```python
from build123d import *

# Parameters (mm, degrees)
EXTRUDE_1_DEPTH     = 14.999999999999998
CUT_EXTRUDE_1_DEPTH = 32.759958749611776
CUT_EXTRUDE_2_DEPTH = 5.999999999999998
CUT_EXTRUDE_START   = -2.9999999999999996
CUT_EXTRUDE_3_DEPTH = 2.9999999999999996
CUT_EXTRUDE_START_2 = -3.0000000000000004
CUT_EXTRUDE_4_DEPTH = 3.0000000000000004
CUT_EXTRUDE_5_DEPTH = 10.50007039461797
CUT_EXTRUDE_6_DEPTH = 11.327672160759418
EXTRUDE_2_DEPTH     = 7.968709711177614
EXTRUDE_3_DEPTH     = 3.000000000000002
HOLE_WIZARD_1_D     = 4.2
HOLE_WIZARD_1_DEPTH = 7
HOLE_WIZARD_2_D     = 2.03
HOLE_WIZARD_2_DEPTH = 4
HOLE_WIZARD_3_D     = 2.03
HOLE_WIZARD_3_DEPTH = 4
HOLE_WIZARD_4_D     = 5.05
HOLE_WIZARD_5_D     = 5.02
HOLE_WIZARD_5_DEPTH = 12
FILLET_1_R          = 5.500000000000002
FILLET_2_R          = 8
CHAMFER_1_SIZE      = 0.9999999999999993
FILLET_3_R          = 0.5


with BuildPart() as part:
    # 草图1 → 凸台-拉伸1 (new body)
    with BuildSketch(Plane(origin=(0, 18, 0), x_dir=(1, 0, 0), z_dir=(0, 1, 0))):
        with BuildLine():
            Line((-17.618889211708797, -12.26572898251346), (21.661848401793918, 2.0312902888225244))
            Line((21.661848401793918, 2.0312902888225244), (-10.5, 2.0312902888223876))
            Line((-10.5, 2.0312902888223876), (-21.381110788291235, -1.9291101538684705))
            ThreePointArc((-21.381110788291235, -1.9291101538684705), (-24.668309414322497, -8.978530356482176), (-17.618889211708797, -12.26572898251346))
        make_face()
    extrude(amount=-EXTRUDE_1_DEPTH)

    # 草图2 → 切除-拉伸1 (cut, through all)
    with BuildSketch(Plane(origin=(0, 18, 0), x_dir=(-1, 0, 0), z_dir=(0, 1, 0))):
        Polygon((-21.66184840179392, -2.0312902888223894), (-5.5000000000000036, -2.0312902888223876), (-5.500000000000005, 3.8511414601534057), align=None)
    extrude(amount=-CUT_EXTRUDE_1_DEPTH, mode=Mode.SUBTRACT)

    # 草图3 → 切除-拉伸2 (cut)
    with BuildSketch(Plane(origin=(0, 18, 0), x_dir=(-1, 0, 0), z_dir=(0, 1, 0))):
        with BuildLine():
            Line((20.78257553747125, 3.5735722402438013), (24.563305918164147, 4.949645562601932))
            ThreePointArc((24.563305918164147, 4.949645562601932), (24.047293898775088, 10.191303567012326), (19.3611131717343, 12.59566569299606))
            Line((19.3611131717343, 12.59566569299606), (20.01010960022055, 10.812562660423456))
            ThreePointArc((20.01010960022055, 10.812562660423456), (15.771169677152303, 6.6995195513380725), (20.78257553747125, 3.5735722402438013))
        make_face()
    extrude(amount=-CUT_EXTRUDE_2_DEPTH, mode=Mode.SUBTRACT)

    # 草图4 → 切除-拉伸3 (cut)
    with BuildSketch(Plane.XZ.offset(-12).offset(CUT_EXTRUDE_START)):
        with BuildLine():
            Line((-20.78257553747125, 3.573572240243805), (-18.036485631419698, 2.5740772538221752))
            Line((-18.036485631419698, 2.5740772538221752), (-17.557657430763733, 3.889646922922488))
            ThreePointArc((-17.557657430763733, 3.889646922922488), (-19.134214632183554, 3.365302064053206), (-20.78257553747125, 3.573572240243805))
        make_face()
    extrude(amount=CUT_EXTRUDE_3_DEPTH, mode=Mode.SUBTRACT)

    # 草图5 → 切除-拉伸4 (cut)
    with BuildSketch(Plane.XZ.offset(-3.000000000000001).offset(CUT_EXTRUDE_START_2)):
        with BuildLine():
            Line((-17.258794358827192, 2.29102077914986), (-16.779966158171227, 3.606590448250214))
            Line((-16.779966158171227, 3.606590448250214), (-17.557657430763737, 3.8896469229224904))
            ThreePointArc((-17.557657430763737, 3.8896469229224904), (-15.965242102135065, 8.349612286378331), (-20.01010960022055, 10.81256266042346))
            Line((-20.01010960022055, 10.81256266042346), (-19.3611131717343, 12.59566569299606))
            ThreePointArc((-19.3611131717343, 12.59566569299606), (-24.04729389877508, 10.191303567012337), (-24.56330591816415, 4.94964556260195))
            Line((-24.56330591816415, 4.94964556260195), (-17.258794358827192, 2.29102077914986))
        make_face()
    extrude(amount=CUT_EXTRUDE_4_DEPTH, mode=Mode.SUBTRACT)

    # 草图6 → 切除-拉伸5 (cut)
    with BuildSketch(Plane(origin=(-15.97621882135595, 0, 5.8148681070970145), x_dir=(0.3420201433256677, 0, 0.9396926207859088), z_dir=(-0.9396926207859089, 0, 0.3420201433256677))):
        Polygon((-2.3499999999999055, 3), (-2.349999999999906, 6), (-3.7499999999999933, 6), (-3.749999999999994, 3), align=None)
    extrude(amount=-CUT_EXTRUDE_5_DEPTH, mode=Mode.SUBTRACT)

    # 草图7 → 切除-拉伸6 (cut)
    with BuildSketch(Plane(origin=(-16.753910093948367, 0, 6.097924581769449), x_dir=(0.3420201433256676, 0, 0.9396926207859088), z_dir=(-0.9396926207859088, 0, 0.3420201433256676))):
        Polygon((-3.749999999999993, 12), (-2.3499999999999055, 12), (-2.3499999999999055, 15), (-3.7499999999999933, 15), align=None)
    extrude(amount=-CUT_EXTRUDE_6_DEPTH, mode=Mode.SUBTRACT)

    # 草图8 → 凸台-拉伸2 (add)
    with BuildSketch(Plane(origin=(-8.63e-15, 0, -2.0312902888224325), x_dir=(-1, 0, 5e-17), z_dir=(-5e-17, 0, -1))):
        Polygon((-5.5, 3), (-5.500000000000001, 18), (10.5, 18), (10.5, 3), align=None)
    extrude(amount=EXTRUDE_2_DEPTH)

    # 草图9 → 凸台-拉伸3 (add)
    with BuildSketch(Plane.XZ.offset(-3.000000000000001)):
        with BuildLine():
            Line((-17.618889211708797, 12.26572898251346), (5.499999999999998, 3.8511414601533294))
            Line((5.499999999999998, 3.8511414601533294), (5.5, -10))
            Line((5.5, -10), (-10.5, -10.000000000000002))
            Line((-10.5, -10.000000000000002), (-10.500000000000014, -2.0312902888224262))
            Line((-10.500000000000014, -2.0312902888224262), (-21.381110788291203, 1.9291101538684652))
            ThreePointArc((-21.381110788291203, 1.9291101538684652), (-23.286441520356178, 3.1083268627098155), (-24.563305918164144, 4.94964556260193))
            Line((-24.563305918164144, 4.94964556260193), (-20.78257553747125, 3.573572240243805))
            ThreePointArc((-20.78257553747125, 3.573572240243805), (-15.771169677152304, 6.699519551338072), (-20.01010960022055, 10.81256266042346))
            Line((-20.01010960022055, 10.81256266042346), (-19.361113171734285, 12.595665692996059))
            ThreePointArc((-19.361113171734285, 12.595665692996059), (-18.476617299855562, 12.50137070130135), (-17.618889211708797, 12.26572898251346))
        make_face()
    extrude(amount=EXTRUDE_3_DEPTH)

    # 孔1
    with Locations(Plane(origin=(-5.4e-16, 0, -10.000000000000046), x_dir=(-1, 0, 5e-17), z_dir=(-5e-17, 0, -1))):
        with Locations((4.5, 9)):
            Hole(HOLE_WIZARD_1_D / 2, depth=HOLE_WIZARD_1_DEPTH)

    # 孔2
    with Locations(Plane(origin=(-5.4e-16, 0, -10.000000000000046), x_dir=(-1, 0, 5e-17), z_dir=(-5e-17, 0, -1))):
        with Locations((-0.5, 13)):
            Hole(HOLE_WIZARD_2_D / 2, depth=HOLE_WIZARD_2_DEPTH)

    # 孔3
    with Locations(Plane(origin=(-5.4e-16, 0, -10.000000000000046), x_dir=(-1, 0, 5e-17), z_dir=(-5e-17, 0, -1))):
        with Locations((-0.5, 5)):
            Hole(HOLE_WIZARD_3_D / 2, depth=HOLE_WIZARD_3_DEPTH)

    # 孔4 (through all)
    with Locations(Plane(origin=(0, 18, 0), x_dir=(1, 0, 0), z_dir=(0, 1, 0))):
        with Locations((-2.585532826, -0.941056988)):
            Hole(HOLE_WIZARD_4_D / 2)

    # 孔5
    with Locations(Plane(origin=(0, 12, 0), x_dir=(1, 0, 0), z_dir=(0, 1, 0))):
        with Locations((-19.5, -7.097419568)):
            Hole(HOLE_WIZARD_5_D / 2, depth=HOLE_WIZARD_5_DEPTH)

    # 圆角1
    fillet_1_edges = [part.edges().sort_by_distance(p)[0] for p in [
        (5.500000000000002, 8.999999999999998, 3.8511414601533676),
    ]]
    fillet(fillet_1_edges, radius=FILLET_1_R)

    # 圆角2
    fillet_2_edges = [part.edges().sort_by_distance(p)[0] for p in [
        (-10.50000000000001, 9, -2.031290288822418),
    ]]
    fillet(fillet_2_edges, radius=FILLET_2_R)

    # 倒角1
    chamfer_1_edges = [part.edges().sort_by_distance(p)[0] for p in [
        (-18.47661729985556, -1.33e-15, 12.50137070130135),
        (-23.286441520356178, -1.33e-15, 3.108326862709817),
        (-18.572474820842935, -1.33e-15, 0.9068502628278257),
        (5.499999999999999, -1.33e-15, -5.000000000000032),
        (-7.868889211708797, -1.33e-15, 8.717019198417944),
        (4.505336243589472, 17.999999999999986, 3.15467039993076),
        (4.505336243589466, -1.65e-14, 3.154670399930683),
        (-10.500000000000002, -1.33e-15, -8.816475297250042),
        (-18.57247482084295, 18, 0.9068502628278368),
        (-11.946783645688074, 17.999999999999993, -3.044339103691696),
        (-11.946783645688082, -7.42e-15, -3.0443391036917093),
        (5.4999999999999964, 18, -5.000000000000016),
        (-18.476617299855565, 18, 12.501370701301362),
        (-7.868889211708806, 18, 8.717019198417947),
        (-23.286441520356195, 18, 3.1083268627098226),
        (-10.500000000000009, 18, -8.816475297250054),
    ]]
    chamfer(chamfer_1_edges, length=CHAMFER_1_SIZE)

    # 圆角3
    fillet_3_edges = [part.edges().sort_by_distance(p)[0] for p in [
        (-14.087265614371681, 3.0000000000000004, 1.1366787190484136),
        (-14.087265614371635, 15, 1.1366787190484962),
        (-15.977630804718132, 6.000000000000001, 1.8247153802274876),
        (-12.23539246068994, 6.000000000000001, 1.9525008949379346),
        (-12.23539246068994, 3.0000000000000004, 1.9525008949379348),
        (-12.235392460689857, 15, 1.952500894938097),
        (-12.235392460689857, 12, 1.952500894938097),
    ]]
    fillet(fillet_3_edges, radius=FILLET_3_R)


solid = part.part
```
The model under review builds one solid part; all positions refer to its coordinate system, in mm. A direction names the side the tool comes from. Coordinates: 2 decimals unless noted, no trailing zeros. Order: outer loops, then holes, each group sorted by start corner. A loop starts at its lowest first (then second) coordinate and runs counter-clockwise, first axis right, second up. Notation, with made-up numbers: (23.25, -29) -> (59.25, -29) arc R21 cw to (59.25, -8) -> close; hole circle Ø9 at (45, 45). An arc over 180 degrees is marked (long way). Answer in a Markdown table with one row per item. Add a question column.
Item 1: We need section B-B on x = -4.5. Write out the cut boundary in (y, z), plus the area to 3 significant figures.
Item 2: We need section A-A on y = 10. Write out the cut boundary in (x, z) (3 decimals).
Item 3: Mouldability with a two-part tool opening along X and no side actions: class faces 1 (the flat face through (-17, 12, 6)), 2 (the flat face through (-5, 9, -3)), 3 (the cylindrical face through (-25, 9, 7)), 4 (the cylindrical face through (-11.91, 9.11, -3.1)) as +X half, -X half, draft (parallel to the pull), parting line (faces both ways), or undercut.
Item 4: Machinability: for faces 5 (the flat face through (-10, 0.5, -8.8)), 6 (the flat face through (-10, 17.5, -8.8)), 7 (the cylindrical face through (0.28, 12.01, -7.97)), which of the approach directions +Z, -Z, +X, -X, +Y, -Y give a long, thin tool a straight path to every point of the face, cutting with its end or side? Answer none if there is none.
Item 5: We need section C-C on y = 5. Write out the cut boundary in (x, z) (3 decimals).
Item 6: Clearance check with flat-ended pins moving along their axes: pin 1 (4.5 mm diameter, centred on x = -4, y = 8.5, fed in from -Z); pin 2 (1.9 mm diameter, centred on y = 5.5, z = -9, fed in from -X); pin 3 (1.6 mm diameter, centred on x = 0.5, y = 13, fed in from +Z); pin 4 (3.5 mm diameter, centred on x = -4.5, y = 9, fed in from +Z). State where each tip first meets the part, or that it passes through.
Item 7: To check wall thickness, follow probe 1 along Y at (x, z) = (-15.5, 2.5); probe 2 along Y at (x, z) = (0.5, -7.15) (3 decimals); probe 3 along Y at (x, z) = (-4.5, -4.5). State the ranges of each line that lie inside material, in increasing order.
Item 8: We need section D-D on x = 1. Write out the cut boundary in (y, z), plus the area to 3 significant figures.
Final values:
| question | item | result |
|---|---|---|
| 1 | outline | (0, -10) -> (6.9, -10) -> (6.9, -3) -> (11.1, -3) -> (11.1, -10) -> (18, -10) -> (18, -0.71) -> (0, -0.71) -> close; (0, 2.59) -> (18, 2.59) -> (18, 6.43) -> (17, 7.49) -> (1, 7.49) -> (0, 6.43) -> close |
| 1 | area | 225 mm2 |
| 2 | outline | (-21.381, 1.929) -> (-15.764, -0.115) arc R8 cw to (-10.5, -7.633) -> (-10.5, -10) -> (-6.347, -10) -> (-6.347, -3) -> (-2.653, -3) -> (-2.653, -10) -> (5.5, -10) -> (5.5, 0) arc R5.5 ccw to (1.881, 5.168) -> (-17.619, 12.266) arc R5.5 ccw to start; hole circle Ø5.02 at (-19.5, 7.097); hole circle Ø5.05 at (-2.586, 0.941) |
| 3 | face 1 | undercut |
| 3 | face 2 | undercut |
| 3 | face 3 | parting line |
| 3 | face 4 | -X half |
| 4 | face 5 | -Z, -X, -Y |
| 4 | face 6 | -Z, -X, +Y |
| 4 | face 7 | -Z |
| 5 | outline | (-24.563, 4.95) arc R5.5 ccw to (-21.381, 1.929) -> (-15.764, -0.115) arc R8 cw to (-10.5, -7.633) -> (-10.5, -10) -> (-0.515, -10) -> (-0.515, -6) -> (1.515, -6) -> (1.515, -10) -> (5.5, -10) -> (5.5, 0) arc R5.5 ccw to (1.881, 5.168) -> (-17.619, 12.266) arc R5.5 ccw to (-19.361, 12.596) -> (-20.01, 10.813) arc R3.75 cw to (-17.558, 3.89) -> (-6.913, 0.015) -> (-7.392, -1.3) -> close; hole circle Ø5.05 at (-2.586, 0.941) |
| 6 | pin 1 | stops at z = -10 |
| 6 | pin 2 | stops at x = -10.5 |
| 6 | pin 3 | stops at z = 5.96 |
| 6 | pin 4 | stops at z = 8.13 |
| 7 | probe 1 | y = 0 to 3, 6 to 12, 15 to 18 |
| 7 | probe 2 | y = 0 to 3.985, 6.015 to 11.985, 14.015 to 18 |
| 7 | probe 3 | y = 0 to 6.9, 11.1 to 18 |
| 8 | outline | (0, -10) -> (4.12, -10) -> (4.12, -6) -> (5.88, -6) -> (5.88, -10) -> (12.12, -10) -> (12.12, -6) -> (13.88, -6) -> (13.88, -10) -> (18, -10) -> (18, 4.42) -> (17, 5.49) -> (1, 5.49) -> (0, 4.42) -> close |
| 8 | area | 264 mm2 |
